Build history of the part. All positions in model axes, mm. A direction names the side the tool comes from. Coordinates: 2 decimals unless noted, no trailing zeros. Order: outer loops, then holes, each group sorted by start corner. A loop starts at its lowest first (then second) coordinate and runs counter-clockwise, first axis right, second up. Notation, with made-up numbers: (52.5, 89.25) -> (103.5, 89.25) arc R24 ccw to (103.5, 115.25) -> close; hole circle Ø9 at (-36.75, -33.75). An arc over 180 degrees is marked (long way). Write each question's results on one line, items separated by ' | '.
from build123d import *

# Parameters (mm, degrees)
SKETCH1_W           = 150
SKETCH1_H           = 130
SKETCH1_R           = 2.500000001
SKETCH1_R_2         = 2
BOSS_EXTRUDE1_DEPTH = 5


with BuildPart() as part:
    # Sketch1 → Boss-Extrude1 (new body)
    with BuildSketch(Plane(origin=(0, 0, 0), x_dir=(1, 0, 0), z_dir=(0, 1, 0))):
        Rectangle(SKETCH1_W, SKETCH1_H)
        with Locations(Location((-15.000000001, 0, 0), (0, 0, 270))):
            Circle(SKETCH1_R, mode=Mode.SUBTRACT)
        with Locations(Location((-30.000000001, 0, 0), (0, 0, 270))):
            Circle(SKETCH1_R, mode=Mode.SUBTRACT)
        with Locations(Location((-60, -15, 0), (0, 0, 270))):
            Circle(SKETCH1_R_2, mode=Mode.SUBTRACT)
        with Locations(Location((-60, -48.737765205, 0), (0, 0, 270))):
            Circle(SKETCH1_R_2, mode=Mode.SUBTRACT)
        with Locations(Location((-27, -48.737765205, 0), (0, 0, 270))):
            Circle(SKETCH1_R_2, mode=Mode.SUBTRACT)
        with Locations(Location((-27, -15, 0), (0, 0, 270))):
            Circle(SKETCH1_R_2, mode=Mode.SUBTRACT)
        with Locations(Location((-27, 15, 0), (0, 0, 270))):
            Circle(SKETCH1_R_2, mode=Mode.SUBTRACT)
        with Locations(Location((-60, 15, 0), (0, 0, 270))):
            Circle(SKETCH1_R_2, mode=Mode.SUBTRACT)
        with Locations(Location((-60, 48.737765205, 0), (0, 0, 270))):
            Circle(SKETCH1_R_2, mode=Mode.SUBTRACT)
        with Locations(Location((-27, 48.737765205, 0), (0, 0, 270))):
            Circle(SKETCH1_R_2, mode=Mode.SUBTRACT)
        with BuildLine():
            Line((0.750570036, -7.209476205), (-10.305683507, -7.209476205))
            Line((-10.305683507, -7.209476205), (-10.305683507, 7.209476205))
            Line((-10.305683507, 7.209476205), (0.750570036, 7.209476205))
            ThreePointArc((0.750570036, 7.209476205), (70, 0), (0.750570036, -7.209476205))
        make_face(mode=Mode.SUBTRACT)
    extrude(amount=BOSS_EXTRUDE1_DEPTH)


solid = part.part
Item 1: Drill centre lines: line 1 (Z direction, x = -4, y = 2.85); line 2 (X direction, y = 1.6, z = -2); line 3 (X direction, y = 1.4, z = 18). Where is each one in solid material? Low to high. Write a range as from..to.
Answer:
line 1: z = -65..-7.21, 7.21..65 | line 2: x = -75..-31.5, -28.5..-16.5, -13.5..-10.31, 69.94..75 | line 3: x = -75..4.98, 65.02..75
Item 2: Slice it at B-B, the plane y = 1.6. State how many separate pieces and enclosed holes the cut face has, and give its area (3 significant figures).
Answer:
separate pieces: 1 | enclosed holes: 11 | area: 15,400 mm^2
Item 3: Pull direction X, two halves, no side cores. Call faces 1 (the cylindrical face through (-58.314, 2.465, -47.663)), 2 (the flat face through (75, 2, 1)), 3 (the flat face through (-18, 5, -1)): released by +X, released by -X, zero draft, split by the parting line, or undercut.
Answer:
face 1: undercut | face 2: released by +X | face 3: zero draft
Item 4: Slice it at A-A, the plane z = -28. List the corners of the cut face in (x, y), and give its area (3 significant figures).
Answer:
outline: (-75, 0) -> (14, 0) -> (14, 5) -> (-75, 5) -> close; (56, 0) -> (75, 0) -> (75, 5) -> (56, 5) -> close | area: 540 mm^2
Item 5: Slice it at C-C, the plane x = 35. List the corners of the cut face in (y, z), and give its area (3 significant figures).
Answer:
outline: (0, -65) -> (5, -65) -> (5, -35) -> (0, -35) -> close; (0, 35) -> (5, 35) -> (5, 65) -> (0, 65) -> close | area: 300 mm^2
Item 6: Slice it at D-D, the plane z = 0. List the corners of the cut face in (x, y), and give its area (3 significant figures).
Answer:
outline: (-75, 0) -> (-32.5, 0) -> (-32.5, 5) -> (-75, 5) -> close; (-27.5, 0) -> (-17.5, 0) -> (-17.5, 5) -> (-27.5, 5) -> close; (-12.5, 0) -> (-10.31, 0) -> (-10.31, 5) -> (-12.5, 5) -> close; (70, 0) -> (75, 0) -> (75, 5) -> (70, 5) -> close | area: 298 mm^2
Item 7: Pin check, flat tip, straight feed: pin 1 (2.5 mm diameter, centred on x = -60, z = -48.74, fed in from +Y). Stop position of the tip, or through.
Answer:
pin 1: passes through
Item 8: Tool access for faces 4 (the flat face through (-5, 2, 7.209)), 5 (the flat face through (-1, 2, -65)): list every direction of +Z, -Z, +X, -X, +Y, -Y with a clear straight run to the whole face (end or side of a thin tool).
Answer:
face 4: +Y, -Y | face 5: -Z, +X, -X, +Y, -Y
